```python
from build123d import *

# Parameters (mm, degrees)
F0_W      = 203.2
F0_H      = 50.8
F1_DEPTH  = 50.8
F2_W      = 38.1
F2_H      = 38.1
F3_DEPTH  = 50.801
F4_DEPTH  = 50.801
F5_W      = 101.6
F5_H      = 25.4
F6_DEPTH  = 38.1
F7_W      = 31.75
F7_H      = 25.4
F7_W_2    = 38.1
F8_DEPTH  = 38.1
F10_DEPTH = 101.601
F12_DEPTH = 50.801
F14_DEPTH = 76.2
F16_START = -25.4
F16_DEPTH = 25.4


with BuildPart() as f1:
    # F0 (on Front) → F1 (new body, symmetric)
    with BuildSketch(Plane.XZ):
        with Locations((101.6, 25.4)):
            Rectangle(F0_W, F0_H)
    extrude(amount=F1_DEPTH, both=True)

    # F2 (on face) → F3 (cut, through all)
    with BuildSketch(Plane.XY.offset(50.8)):
        with Locations((184.15, 0)):
            Rectangle(F2_W, F2_H)
    extrude(amount=-F3_DEPTH, mode=Mode.SUBTRACT)

    # F2 (on face) → F4 (cut, through all)
    with BuildSketch(Plane.XY.offset(50.8)):
        with Locations((19.05, 0)):
            Rectangle(F2_W, F2_H)
    extrude(amount=-F4_DEPTH, mode=Mode.SUBTRACT)

    # F5 (on Right) → F6 (cut)
    with BuildSketch(Plane.YZ):
        with Locations((0, 12.7)):
            Rectangle(F5_W, F5_H)
    extrude(amount=F6_DEPTH, mode=Mode.SUBTRACT)

    # F7 (on face) → F8 (cut)
    with BuildSketch(Plane.YZ.offset(165.1)):
        with Locations((34.925, 12.7)):
            Rectangle(F7_W, F7_H)
        with Locations((0, 12.7)):
            Rectangle(F7_W_2, F7_H)
        with Locations((-34.925, 12.7)):
            Rectangle(F7_W, F7_H)
    extrude(amount=F8_DEPTH, mode=Mode.SUBTRACT)

    # F9 (on face) → F10 (cut, through all)
    with BuildSketch(Plane.XZ.offset(50.8)):
        with BuildLine():
            Line((63.5, 19.0500015557), (63.5, 0))
            Line((63.5, 0), (139.7, 0))
            Line((139.7, 0), (139.7, 19.0500015557))
            ThreePointArc((139.7, 19.0500015557), (137.8401280605, 23.5401296162), (133.35, 25.4000015557))
            Line((133.35, 25.4000015557), (69.85, 25.4000015557))
            ThreePointArc((69.85, 25.4000015557), (65.3598719395, 23.5401296162), (63.5, 19.0500015557))
        make_face()
    extrude(amount=-F10_DEPTH, mode=Mode.SUBTRACT)

    # F11 (on face) → F12 (cut, through all)
    with BuildSketch(Plane.XY.offset(50.8)):
        with BuildLine():
            Line((0, 50.8), (0, 38.1))
            ThreePointArc((0, 38.1), (3.7197438789, 47.0802561211), (12.7, 50.8))
            Line((12.7, 50.8), (0, 50.8))
        make_face()
        with BuildLine():
            Line((0, -50.8), (12.7, -50.8))
            ThreePointArc((12.7, -50.8), (3.7197438789, -47.0802561211), (0, -38.1))
            Line((0, -38.1), (0, -50.8))
        make_face()
        with BuildLine():
            ThreePointArc((203.2, -38.1), (199.4802561211, -47.0802561211), (190.5, -50.8))
            Line((190.5, -50.8), (203.2, -50.8))
            Line((203.2, -50.8), (203.2, -38.1))
        make_face()
        with BuildLine():
            ThreePointArc((190.5, 50.8), (199.4802561211, 47.0802561211), (203.2, 38.1))
            Line((203.2, 38.1), (203.2, 50.8))
            Line((203.2, 50.8), (190.5, 50.8))
        make_face()
    extrude(amount=-F12_DEPTH, mode=Mode.SUBTRACT)

    # F13 (on face) → F14 (join)
    with BuildSketch(Plane.XY.offset(50.8)):
        Polygon((152.4, 50.8), (50.8, 50.8), (101.6, -50.8), align=None)
    extrude(amount=F14_DEPTH)

    # F15 (on face) → F16 (cut)
    with BuildSketch(Plane.XY.offset(127).offset(F16_START)):
        Polygon((101.6, -50.8), (127, 0), (76.2, 0), align=None)
    extrude(amount=-F16_DEPTH, mode=Mode.SUBTRACT)


solid = f1.part
```
Model file for the job. Use its own axes, mm. A direction names the side the tool comes from. Coordinates: 2 decimals unless noted, no trailing zeros. Order: outer loops, then holes, each group sorted by start corner. A loop starts at its lowest first (then second) coordinate and runs counter-clockwise, first axis right, second up. Notation, with made-up numbers: (0.25, -40) - (41.25, -40) arc R18 cw to (41.25, -32) - close; hole circle Ø2 at (65, 68). An arc over 180 degrees is marked (long way). Return JSON: item names as keys, results as strings. Group by question number.
1) Saw through at A-A, the plane y = -35.5. Write the cut outline in (x, z).
2) Saw through at D-D, the plane z = 27.5. Write the cut outline in (x, y).
3) Probe line 1 (Z direction, x = 101.5, y = -17.5); line 2 (Z direction, x = 82.5, y = 31); line 3 (X direction, y = -8.5, z = 30). List the from-to ranges inside material, lowest first. Write a range as from..to.
4) Saw through at C-C, the plane y = 16.5. Write the cut outline in (x, z).
5) Mould opens along Y. For faces 1 (the flat face through (132.3, 10.6, 88.4)), 2 (the flat face through (184, -19.05, 38)), 3 (the cylindrical face through (199.38, 47.18, 38.28)) say: released by +Y, released by -Y, zero draft, split by the parting line, or undercut.
6) Tool access for faces 4 (the flat face through (101, -19, 76.2)), 5 (the flat face through (63.5, -1, 10)), 6 (the flat face through (163, -12, 50.8)), 7 (the flat face through (75.844, 0.711, 88.367)): list every direction of +Z, -Z, +X, -X, +Y, -Y with a clear straight run to the whole face (end or side of a thin tool).
7) Flat gauge pins, fed straight in: P1, Ø12.5, axis at x = 101.5, z = 85.5, coming from the -Y side; P2, Ø3, axis at y = -16.5, z = 62.5, coming from the -X side; P3, Ø10, axis at y = -27, z = 20, coming from the -X side. Where does each tip first touch, or does it go through?
8) Saw through at B-B, the plane x = 176.5. Write the cut outline in (y, z), plus the area to 3 significant figures.
Values found:
{
 "1": {"outline": "(0, 25.4) - (38.1, 25.4) - (38.1, 0) - (63.5, 0) - (63.5, 19.05) arc R6.35 cw to (69.85, 25.4) - (133.35, 25.4) arc R6.35 cw to (139.7, 19.05) - (139.7, 0) - (165.1, 0) - (165.1, 25.4) - (203.2, 25.4) - (203.2, 50.8) - (109.25, 50.8) - (109.25, 76.2) - (93.95, 76.2) - (93.95, 50.8) - (0, 50.8) - close; (93.95, 101.6) - (109.25, 101.6) - (109.25, 127) - (93.95, 127) - close"},
 "2": {"outline": "(0, -38.1) arc R12.7 ccw to (12.7, -50.8) - (190.5, -50.8) arc R12.7 ccw to (203.2, -38.1) - (203.2, -19.05) - (165.1, -19.05) - (165.1, 19.05) - (203.2, 19.05) - (203.2, 38.1) arc R12.7 ccw to (190.5, 50.8) - (12.7, 50.8) arc R12.7 ccw to (0, 38.1) - (0, 19.05) - (38.1, 19.05) - (38.1, -19.05) - (0, -19.05) - close"},
 "3": {"line 1": "z = 25.4..76.2, 101.6..127", "line 2": "z = 25.4..127", "line 3": "x = 38.1..165.1"},
 "4": {"outline": "(38.1, 0) - (63.5, 0) - (63.5, 19.05) arc R6.35 cw to (69.85, 25.4) - (133.35, 25.4) arc R6.35 cw to (139.7, 19.05) - (139.7, 0) - (165.1, 0) - (165.1, 50.8) - (135.25, 50.8) - (135.25, 127) - (67.95, 127) - (67.95, 50.8) - (38.1, 50.8) - close"},
 "5": {"face 1": "released by -Y", "face 2": "undercut", "face 3": "released by +Y"},
 "6": {"face 4": "+X, -X, -Y", "face 5": "-Z, +Y, -Y", "face 6": "+Z, +X, -Y", "face 7": "+Z, -X, -Y"},
 "7": {"P1": "stops at y = 0", "P2": "stops at x = 83.7", "P3": "stops at x = 38.1"},
 "8": {"outline": "(-50.8, 25.4) - (-19.05, 25.4) - (-19.05, 50.8) - (-50.8, 50.8) - close; (19.05, 25.4) - (50.8, 25.4) - (50.8, 50.8) - (19.05, 50.8) - close", "area": "1,610 mm²"}
}
